Verification items for this drawing (mm, ordinates from the low corner). A direction names the side the tool comes from. Coordinates: 2 decimals unless noted, no trailing zeros. Order: outer loops, then holes, each group sorted by start corner. A loop starts at its lowest first (then second) coordinate and runs counter-clockwise, first axis right, second up. Notation, with made-up numbers: M -39.5,56.5 L -26.5,56.5 A12 cw -26.5,64.5 Z; hole C -28.75,80.25 d4. An arc over 180 degrees is marked long. Answer as a JSON object with one key per item and string values. Group by question number.
(1) Access from +Z, -Z, +X, -X, +Y, -Y to the whole of each face (thin tool, end or side, straight path). Record for the marked faces 5 and 6.
(2) Material ranges on line 1 (Y direction, x = 2.25, z = 0.7) (1 decimal); line 2 (Y direction, x = 4, z = 1.8) (1 decimal); line 3 (X direction, y = 2.25, z = 2.2) (1 decimal), recorded low to high.
(3) Cross-section at A-A (y = 4.34). Enter the section's corners in (x, z), plus the area to 3 significant figures.
(4) Cross-section at D-D (y = 7.75). Enter the section's corners in (x, z) (1 decimal), plus the area to 3 significant figures.
(5) Mould release check, pull along X, two halves, no side actions. Record for the marked faces 1, 2, 3 and 4: released by +X, released by -X, zero draft, split by the parting line, or undercut.
(6) Cross-section at B-B (x = 4.25). Enter the section's corners in (y, z).
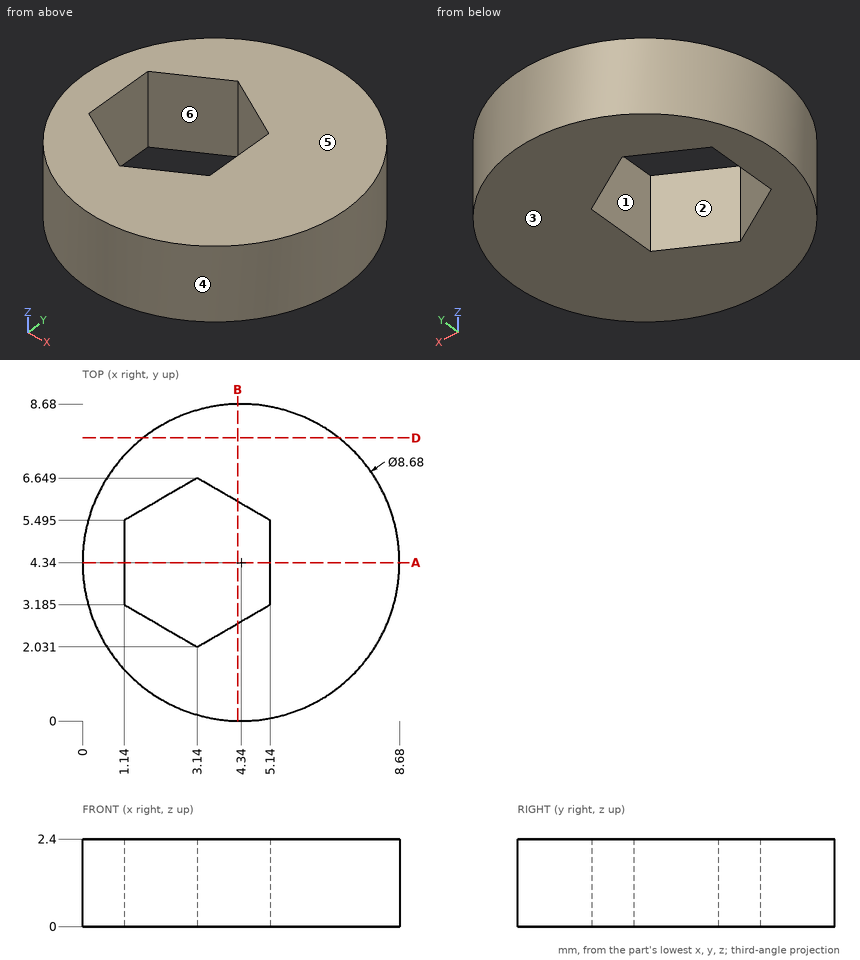
Taken from the geometry:
{
 "1": {"face 5": "+Z, +X, -X, +Y, -Y", "face 6": "+Z, -Z"},
 "2": {"line 1": "y = 0.5 to 2.5, 6.1 to 8.1", "line 2": "y = 0 to 2.5, 6.2 to 8.7", "line 3": "x = 0.5 to 2.8, 3.5 to 8.1"},
 "3": {"outline": "M 0,0 L 1.14,0 L 1.14,2.4 L 0,2.4 Z; M 5.14,0 L 8.68,0 L 8.68,2.4 L 5.14,2.4 Z", "area": "11.2 mm²"},
 "4": {"outline": "M 1.7,0 L 7,0 L 7,2.4 L 1.7,2.4 Z", "area": "12.9 mm²"},
 "5": {"face 1": "undercut", "face 2": "undercut", "face 3": "zero draft", "face 4": "split by the parting line"},
 "6": {"outline": "M 0,0 L 2.67,0 L 2.67,2.4 L 0,2.4 Z; M 6.01,0 L 8.68,0 L 8.68,2.4 L 6.01,2.4 Z"}
}
